```python
from build123d import *

# Parameters (mm, degrees)
BOSS_EXTRUDE1_DEPTH = 15
SKETCH5_R           = 2.5
BOSS_EXTRUDE3_DEPTH = 2.5


with BuildPart() as part:
    # Sketch2 → Boss-Extrude1 (new body, symmetric)
    with BuildSketch(Plane(origin=(0, 0, 0), x_dir=(0, 0, -1), z_dir=(1, 0, 0))):
        Polygon((0, 0), (0, 2530), (890, 2530), (890, 0), (860, 0), (860, 2500), (30, 2500), (30, 0), align=None)
    extrude(amount=BOSS_EXTRUDE1_DEPTH, both=True)

    # Sketch5 → Boss-Extrude3 (add, symmetric)
    with BuildSketch(Plane.XZ):
        with Locations((0, -15)):
            Circle(SKETCH5_R)
        with Locations((0, -875)):
            Circle(SKETCH5_R)
    extrude(amount=BOSS_EXTRUDE3_DEPTH, both=True)


solid = part.part
```
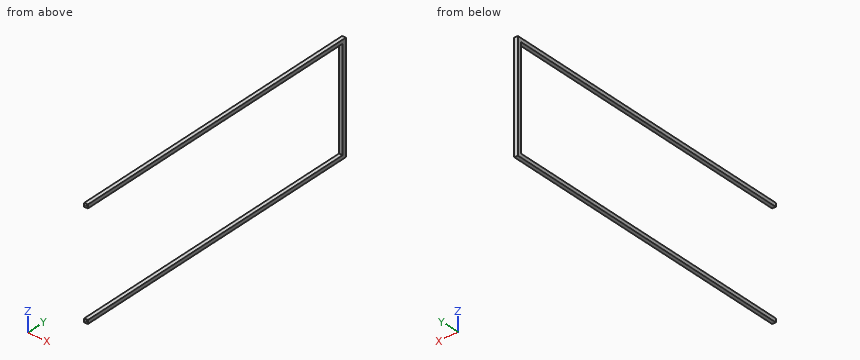
Can you work these out from the model? Positions are in its coordinate system, mm. Give positions to 0.01 mm unless a question says otherwise; leave off trailing zeros. Loops run counter-clockwise (first coordinate to the right, second up) from the corner with the lowest first, then second, coordinate; pieces in that order, holes last. Notation, with made-up numbers: M -12,-29.5 L -7,-29.5 A14 cw -7,-16.5 Z; hole C 55.25,-22.75 d5. An arc over 180 degrees is marked long. One line per question, with ' | ' between items. Start each with the question number.
Q1. If we section it at B-B (z = -718): Please give me the cut outline in (x, y).
Q2. For pin 1 Ø2 at (x, y) = (1.5, 2094) entering from +Z; pin 2 Ø12 at (x, z) = (-10.5, -646.5) entering from -Y, each with a flat end and sliding along its axis, tell me the tip position at first contact or that it passes through.
Q3. If we section it at A-A (y = 1979): Please give me the cut outline in (x, z).
Q4. If I drill on line 1 (Z direction, x = 2.5, y = 1476); line 2 (Y direction, x = 10, z = -168.5), over which ranges is the centre line in solid material (lowest first)? Write a range as from..to.
Computed:
1) outline: M -15,2500 L 15,2500 L 15,2530 L -15,2530 Z
2) pin 1: stops at z = 0 | pin 2: stops at y = 2500
3) outline: M -15,-890 L 15,-890 L 15,-860 L -15,-860 Z; M -15,-30 L 15,-30 L 15,0 L -15,0 Z
4) line 1: z = -890..-860, -30..0 | line 2: y = 2500..2530
